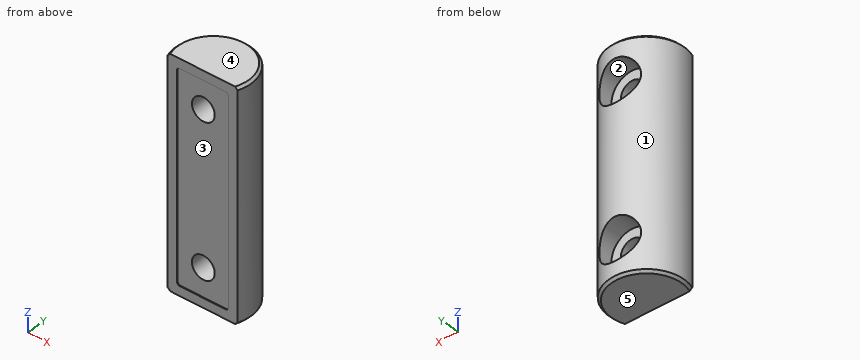
```python
from build123d import *

# Parameters (mm, degrees)
SKETCH1_R            = 6.35
EXTRUDE1_DEPTH       = 19.05
CHAMFER1_SIZE        = 0.4064
TRUNCATED_DEPTH      = 20.05
TRUNCATED_DEPTH_BACK = 20.05
RECESSED_DEPTH       = 0.127


with BuildPart() as part:
    # Sketch1 → Extrude1 (new body, symmetric)
    with BuildSketch(Plane.XY):
        Circle(SKETCH1_R)
    extrude(amount=EXTRUDE1_DEPTH, both=True)

    # Chamfer1
    chamfer1_edges = [part.edges().sort_by_distance(p)[0] for p in [
        (-6.35, 0, -19.05),
        (-6.35, 0, 19.05),
    ]]
    chamfer(chamfer1_edges, length=CHAMFER1_SIZE)

    # Sketch2 → Truncated (cut, two sides)
    with BuildSketch(Plane.XY) as truncated_sk:
        with BuildLine():
            Line((-5.980823609, -2.1336), (5.980823609, -2.1336))
            ThreePointArc((5.980823609, -2.1336), (0, -6.35), (-5.980823609, -2.1336))
        make_face()
    extrude(amount=TRUNCATED_DEPTH, mode=Mode.SUBTRACT)
    extrude(truncated_sk.sketch, amount=-TRUNCATED_DEPTH_BACK, mode=Mode.SUBTRACT)

    # Sketch3 → Recessed (cut)
    with BuildSketch(Plane.XZ.offset(2.1336)):
        with BuildLine():
            Line((3.885323609, 17.4625), (-3.885323609, 17.4625))
            ThreePointArc((-3.885323609, 17.4625), (-4.244533854, 17.313710245), (-4.393323609, 16.9545))
            Line((-4.393323609, 16.9545), (-4.393323609, -16.9545))
            ThreePointArc((-4.393323609, -16.9545), (-4.244533854, -17.313710245), (-3.885323609, -17.4625))
            Line((-3.885323609, -17.4625), (3.885323609, -17.4625))
            ThreePointArc((3.885323609, -17.4625), (4.244533854, -17.313710245), (4.393323609, -16.9545))
            Line((4.393323609, -16.9545), (4.393323609, 16.9545))
            ThreePointArc((4.393323609, 16.9545), (4.244533854, 17.313710245), (3.885323609, 17.4625))
        make_face()
    extrude(amount=-RECESSED_DEPTH, mode=Mode.SUBTRACT)

    # Sketch5 → CtBored Hole Cut-Revolve1 (revolve, cut)
    with BuildSketch(Plane(origin=(0, 0, 0), x_dir=(0, 0, -1), z_dir=(1, 0, 0)), mode=Mode.PRIVATE) as ctbored_hole_cut_revolve1_sk:
        Polygon((14.6558, -6.35), (14.6558, 2.8448), (16.2687, 2.8448), (16.2687, 6.35), (12.7, 6.35), (12.7, -6.35), align=None)
    ctbored_hole_cut_revolve1 = revolve(ctbored_hole_cut_revolve1_sk.sketch.rotate(Axis((0, 11.226654631, -12.7), (0, -1, 0)), 180), axis=Axis((0, 11.226654631, -12.7), (0, -1, 0)), mode=Mode.SUBTRACT)  # turned: the seam where the file's is

    # CtBored Hole Mirror1: CtBored Hole Cut-Revolve1 across plane
    add(ctbored_hole_cut_revolve1.mirror(Plane.XY), mode=Mode.SUBTRACT)


solid = part.part
```
Part model, mm, in its own coordinate system. Face numbers are marked on the shaded views. A direction names the side the tool comes from. Round coordinates to 2 decimals unless told otherwise and drop trailing zeros. Loops run counter-clockwise (first coordinate to the right, second up) from the corner with the lowest first, then second, coordinate; pieces in that order, holes last.
Item 1: Cut at C-C, the plane z = -12.7. Give the cut face in (x, y), then the cut area to 3 significant figures.
Item 2: Drill centre lines: line 1 (Z direction, x = 3, y = 3.5); line 2 (X direction, y = 4.05, z = -12.7); line 3 (X direction, y = 2, z = 11). Where is each one in solid material? Low to high.
Item 3: Cut at A-A, the plane x = 0. Give the cut face in (y, z), then the cut area to 3 significant figures.
Item 4: 3-axis set-ups, long thin cutter, end or side, ignore diameter. For the marked faces 1 and 2: which of +Z, -Z, +X, -X, +Y, -Y reach the whole face in a straight line?
Item 5: Cut at B-B, the plane y = 0. Give the cut face in (x, z).
Item 6: Mould opens along Z. For the marked faces 3, 4 and 5 say: +Z half, -Z half, draft (parallel to the pull), parting line (faces both ways), or undercut.
Item 7: Cut at D-D, the plane z = 8. Give the cut face in (x, y), then the cut area to 3 significant figures.
Item 8: Drop flat-ended pins along their axis: P1, Ø5, axis at x = -3.5, z = 9, coming from the +Y side; P2, Ø5.5, axis at x = 0, z = -12.7, coming from the +Y side; P3, Ø2, axis at y = 2, z = 6.5, coming from the +X side; P4, Ø2.5, axis at x = 0, z = 12.7, coming from the +Y side. Give the stop position or say it passes through.
A:
1. outline: (-5.98, -2.13) - (-4.39, -2.13) - (-4.39, -2.01) - (-1.96, -2.01) - (-1.96, 2.84) - (-3.57, 2.84) - (-3.57, 5.25) arc R6.35 ccw to start; (1.96, -2.01) - (4.39, -2.01) - (4.39, -2.13) - (5.98, -2.13) arc R6.35 ccw to (3.57, 5.25) - (3.57, 2.84) - (1.96, 2.84) - close
1. area: 47.3 mm2
2. line 1: z = -19.05 to -14.63, -10.77 to 10.77, 14.63 to 19.05
2. line 2: x = -4.89 to -3.57, 3.57 to 4.89
2. line 3: x = -6.03 to -0.97, 0.97 to 6.03
3. outline: (-2.13, -19.05) - (5.94, -19.05) - (6.35, -18.64) - (6.35, -16.27) - (2.84, -16.27) - (2.84, -14.66) - (-2.01, -14.66) - (-2.01, -17.46) - (-2.13, -17.46) - close; (-2.13, 17.46) - (-2.01, 17.46) - (-2.01, 14.66) - (2.84, 14.66) - (2.84, 16.27) - (6.35, 16.27) - (6.35, 18.64) - (5.94, 19.05) - (-2.13, 19.05) - close; (-2.01, -10.74) - (2.84, -10.74) - (2.84, -9.13) - (6.35, -9.13) - (6.35, 9.13) - (2.84, 9.13) - (2.84, 10.74) - (-2.01, 10.74) - close
3. area: 231 mm2
4. face 1: +Z, -Z
4. face 2: +Y
5. outline: (-6.35, -18.64) - (-5.94, -19.05) - (5.94, -19.05) - (6.35, -18.64) - (6.35, 18.64) - (5.94, 19.05) - (-5.94, 19.05) - (-6.35, 18.64) - close; hole circle Ø3.91 at (0, -12.7); hole circle Ø3.91 at (0, 12.7)
6. face 3: undercut
6. face 4: +Z half
6. face 5: -Z half
7. outline: (-5.98, -2.13) - (-4.39, -2.13) - (-4.39, -2.01) - (4.39, -2.01) - (4.39, -2.13) - (5.98, -2.13) arc R6.35 ccw (long way) to start
7. area: 88.8 mm2
8. P1: stops at y = 6.27
8. P2: stops at y = 2.84
8. P3: stops at x = 6.27
8. P4: passes through
